Check sheet for the modelled part. Datum: model origin and axes. Units: mm. Face numbers are marked on the shaded views. A direction names the side the tool comes from. Round coordinates to 2 decimals unless told otherwise and drop trailing zeros. Loops run counter-clockwise (first coordinate to the right, second up) from the corner with the lowest first, then second, coordinate; pieces in that order, holes last. Notation, with made-up numbers: (-34, 0.5) - (2, 0.5) arc R18 cw to (2, 11.5) - close; hole circle Ø10 at (41.5, 64.25). An arc over 180 degrees is marked (long way). Answer in a Markdown table with one row per item. Add a question column.
(1) Cross-section at B-B on z = 15.75. Enter the section's corners in (x, y), then the cut area to 3 significant figures.
(2) Access from +Z, -Z, +X, -X, +Y, -Y to the whole of each face (thin tool, end or side, straight path). Record for the marked faces 4, 5, 6, 7 and 8.
(3) Gauge pin test, flat ends, axial feed: pin 1 (8 mm diameter, centred on y = 11, z = 10, fed in from -X) (3 decimals); pin 2 (3 mm diameter, centred on x = -11, y = -0.5, fed in from +Z); pin 3 (4 mm diameter, centred on y = 11, z = 10, fed in from +X). Record the tip position at first contact, or that the pin passes through.
(4) Cross-section at C-C on y = -2.5. Enter the section's corners in (x, z).
(5) Mould release check, pull along Y, two halves, no side actions. Record for the marked faces 1, 2 and 3: +Y half, -Y half, draft (parallel to the pull), parting line (faces both ways), or undercut.
(6) Cross-section at D-D on x = 7.5. Enter the section's corners in (y, z).
(7) Cross-section at A-A on x = -10. Enter the section's corners in (y, z).
(8) Thickness scan on line 1 along Y through (x, z) = (0, 15.5); line 2 along X through (y, z) = (15.5, 7.5); line 3 along Z through (x, y) = (-21.5, 11). Record the ranges inside material, lowest first.
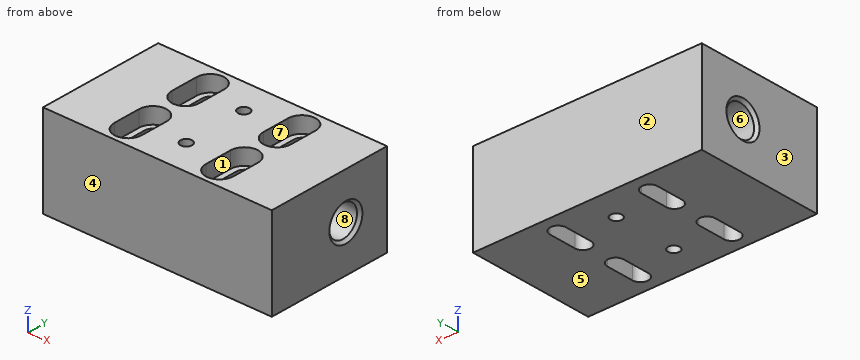
from build123d import *

# Parameters (mm, degrees)
SKETCH1_W             = 50
SKETCH1_H             = 14
BOSS_EXTRUDE1_DEPTH   = 20
CUT_EXTRUDE1_DEPTH    = 3.5
CUT_EXTRUDE2_DEPTH    = 31.761176831
M3X0_5_TAPPED_HOLE1_D = 2.5
MIRROR1_OUTLINE_W     = 50
MIRROR1_OUTLINE_H     = 14
MIRROR1_OUTLINE_R     = 1.25
MIRROR1_DEPTH         = 20
MIRROR1_2_DEPTH       = 16.5


# Read off the part's stored shape, not the designer's step: Mirror1
with BuildPart() as part:
    # Sketch1 → Boss-Extrude1 (new body)
    with BuildSketch(Plane.XY):
        Rectangle(SKETCH1_W, SKETCH1_H)
    extrude(amount=BOSS_EXTRUDE1_DEPTH)

    # Sketch2 → Cut-Extrude1 (cut)
    with BuildSketch(Plane.XY.offset(20)):
        with BuildLine():
            Line((-7, 3), (-7, -3))
            ThreePointArc((-7, -3), (-10, -6), (-13, -3))
            Line((-13, -3), (-13, 3))
            ThreePointArc((-13, 3), (-10, 6), (-7, 3))
        make_face()
        with BuildLine():
            Line((13, 3), (13, -3))
            ThreePointArc((13, -3), (10, -6), (7, -3))
            Line((7, -3), (7, 3))
            ThreePointArc((7, 3), (10, 6), (13, 3))
        make_face()
    extrude(amount=-CUT_EXTRUDE1_DEPTH, mode=Mode.SUBTRACT)

    # Sketch3 → Cut-Extrude2 (cut, through all)
    with BuildSketch(Plane.XY.offset(16.5)):
        with BuildLine():
            Line((-11.75, 3), (-11.75, -3))
            ThreePointArc((-11.75, -3), (-10, -4.75), (-8.25, -3))
            Line((-8.25, -3), (-8.25, 3))
            ThreePointArc((-8.25, 3), (-10, 4.75), (-11.75, 3))
        make_face()
        with BuildLine():
            Line((11.75, -3), (11.75, 3))
            ThreePointArc((11.75, 3), (10, 4.75), (8.25, 3))
            Line((8.25, 3), (8.25, -3))
            ThreePointArc((8.25, -3), (10, -4.75), (11.75, -3))
        make_face()
    extrude(amount=-CUT_EXTRUDE2_DEPTH, mode=Mode.SUBTRACT)

    # M3x0.5 Tapped Hole1 (through all)
    with Locations(Plane.XY.offset(20)):
        with Locations((0, 0)):
            Hole(M3X0_5_TAPPED_HOLE1_D / 2)

    # Mirror1 outline → Mirror1 (add)
    with BuildSketch(Plane.XY):
        with Locations((0, 14)):
            Rectangle(MIRROR1_OUTLINE_W, MIRROR1_OUTLINE_H)
        with BuildLine():
            ThreePointArc((-13, 17), (-10, 20), (-7, 17))
            Line((-7, 17), (-7, 11))
            ThreePointArc((-7, 11), (-10, 8), (-13, 11))
            Line((-13, 11), (-13, 17))
        make_face(mode=Mode.SUBTRACT)
        with Locations((0, 14)):
            Circle(MIRROR1_OUTLINE_R, mode=Mode.SUBTRACT)
        with BuildLine():
            ThreePointArc((7, 17), (10, 20), (13, 17))
            Line((13, 17), (13, 11))
            ThreePointArc((13, 11), (10, 8), (7, 11))
            Line((7, 11), (7, 17))
        make_face(mode=Mode.SUBTRACT)
    extrude(amount=MIRROR1_DEPTH)

    # Mirror1 2 outline → Mirror1 2 (add)
    # profile 1 of 2: a face of its own
    with BuildSketch(Plane.XY):
        with BuildLine():
            Line((13, 11), (13, 17))
            ThreePointArc((13, 17), (10, 20), (7, 17))
            Line((7, 17), (7, 11))
            ThreePointArc((7, 11), (10, 8), (13, 11))
        make_face()
        with BuildLine():
            ThreePointArc((11.75, 11), (10, 9.25), (8.25, 11))
            Line((8.25, 11), (8.25, 17))
            ThreePointArc((8.25, 17), (10, 18.75), (11.75, 17))
            Line((11.75, 17), (11.75, 11))
        make_face(mode=Mode.SUBTRACT)
    # profile 2 of 2: a face of its own
    with BuildSketch(Plane.XY):
        with BuildLine():
            Line((-7, 11), (-7, 17))
            ThreePointArc((-7, 17), (-10, 20), (-13, 17))
            Line((-13, 17), (-13, 11))
            ThreePointArc((-13, 11), (-10, 8), (-7, 11))
        make_face()
        with BuildLine():
            ThreePointArc((-11.75, 17), (-10, 18.75), (-8.25, 17))
            Line((-8.25, 17), (-8.25, 11))
            ThreePointArc((-8.25, 11), (-10, 9.25), (-11.75, 11))
            Line((-11.75, 11), (-11.75, 17))
        make_face(mode=Mode.SUBTRACT)
    extrude(amount=MIRROR1_2_DEPTH)

    # Sketch10 → M8x1.25 Tapped Hole1 (revolve, cut)
    with BuildSketch(Plane(origin=(25, 11, 10), x_dir=(0, 0, -1), z_dir=(0, 1, 0))):
        Polygon((0, 0), (0, 9.75), (3.4, 7.707073895), (3.4, 0.625), (4.025, 0), align=None)
    m8x1_25_tapped_hole1 = revolve(axis=Axis((31.35, 11, 10), (-1, 0, 0)), mode=Mode.SUBTRACT)

    # Mirror2: M8x1.25 Tapped Hole1 across plane
    add(m8x1_25_tapped_hole1.mirror(Plane(origin=(0, 0, 0), x_dir=(0, 0, 1), z_dir=(1, 0, 0))), mode=Mode.SUBTRACT)


solid = part.part
Answers:
| question | item | result |
|---|---|---|
| 1 | outline | (-25, -7) - (25, -7) - (25, 21) - (-25, 21) - close; hole (-11.75, -3) arc R1.75 ccw to (-8.25, -3) - (-8.25, 3) arc R1.75 ccw to (-11.75, 3) - close; hole (-11.75, 11) arc R1.75 ccw to (-8.25, 11) - (-8.25, 17) arc R1.75 ccw to (-11.75, 17) - close; hole circle Ø2.5 at (0, 0); hole circle Ø2.5 at (0, 14); hole (8.25, -3) arc R1.75 ccw to (11.75, -3) - (11.75, 3) arc R1.75 ccw to (8.25, 3) - close; hole (8.25, 11) arc R1.75 ccw to (11.75, 11) - (11.75, 17) arc R1.75 ccw to (8.25, 17) - close |
| 1 | area | 1,270 mm^2 |
| 2 | face 4 | +Z, -Z, +X, -X, -Y |
| 2 | face 5 | -Z, +X, -X, +Y, -Y |
| 2 | face 6 | -X |
| 2 | face 7 | +Z |
| 2 | face 8 | +X |
| 3 | pin 1 | stops at x = -24.975 |
| 3 | pin 2 | stops at z = 16.5 |
| 3 | pin 3 | stops at x = 16.45 |
| 4 | outline | (-25, 0) - (-11.75, 0) - (-11.75, 16.5) - (-13, 16.5) - (-13, 20) - (-25, 20) - close; (-8.25, 0) - (8.25, 0) - (8.25, 16.5) - (7, 16.5) - (7, 20) - (-7, 20) - (-7, 16.5) - (-8.25, 16.5) - close; (11.75, 0) - (25, 0) - (25, 20) - (13, 20) - (13, 16.5) - (11.75, 16.5) - close |
| 5 | face 1 | undercut |
| 5 | face 2 | +Y half |
| 5 | face 3 | draft |
| 6 | outline | (-7, 0) - (21, 0) - (21, 20) - (18.66, 20) - (18.66, 16.5) - (9.34, 16.5) - (9.34, 20) - (4.66, 20) - (4.66, 16.5) - (-4.66, 16.5) - (-4.66, 20) - (-7, 20) - close |
| 7 | outline | (-7, 0) - (-4.75, 0) - (-4.75, 16.5) - (-6, 16.5) - (-6, 20) - (-7, 20) - close; (4.75, 0) - (9.25, 0) - (9.25, 16.5) - (8, 16.5) - (8, 20) - (6, 20) - (6, 16.5) - (4.75, 16.5) - close; (18.75, 0) - (21, 0) - (21, 20) - (20, 20) - (20, 16.5) - (18.75, 16.5) - close |
| 8 | line 1 | y = -7 to -1.25, 1.25 to 12.75, 15.25 to 21 |
| 8 | line 2 | x = -25 to -11.75, -8.25 to 8.25, 11.75 to 25 |
| 8 | line 3 | z = 0 to 6.6, 13.4 to 20 |
